from build123d import *

# Parameters (mm, degrees)
SKETCH_1_W      = 60
SKETCH_1_H      = 18
SKETCH_1_W_2    = 50
SKETCH_1_H_2    = 8
EXTRUDE_1_DEPTH = 50
SKETCH_2_W      = 50
SKETCH_2_H      = 8
EXTRUDE_2_DEPTH = 0.5


with BuildPart() as part:
    # 스케치1 → 보스-돌출1 (new body)
    with BuildSketch(Plane.XY):
        with Locations((25, 4)):
            Rectangle(SKETCH_1_W, SKETCH_1_H)
        with Locations((25, 4)):
            Rectangle(SKETCH_1_W_2, SKETCH_1_H_2, mode=Mode.SUBTRACT)
    extrude(amount=EXTRUDE_1_DEPTH)

    # 스케치2 → 보스-돌출2 (add, symmetric)
    with BuildSketch(Plane.XY.offset(25)):
        with Locations((25, 4)):
            Rectangle(SKETCH_2_W, SKETCH_2_H)
    extrude(amount=EXTRUDE_2_DEPTH, both=True)


solid = part.part
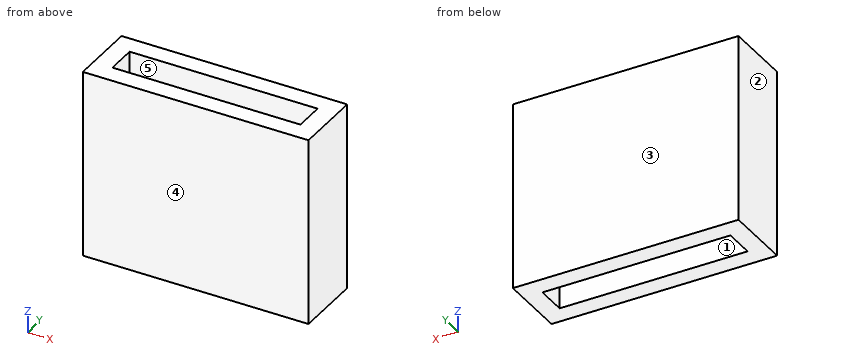
Geometry check sheet. Reference: the model listing, model coordinates, mm. Face numbers are marked on the shaded views. A direction names the side the tool comes from. Round coordinates to 2 decimals unless told otherwise and drop trailing zeros. Loops run counter-clockwise (first coordinate to the right, second up) from the corner with the lowest first, then second, coordinate; pieces in that order, holes last.
Item 1: Cross-section at B-B on y = 5.75. Record the boundary of the cut face in (x, z), then the cut area to 3 significant figures.
Item 2: Cross-section at A-A on z = 10. Record the boundary of the cut face in (x, y).
Item 3: Thickness scan on line 1 (Y direction, x = 45.5, z = 44.5); line 2 (X direction, y = 4, z = 32); line 3 (Z direction, x = 2.5, y = 1.25). Record the ranges inside material, lowest first.
Item 4: Mould release check, pull along Y, two halves, no side actions. Record for the marked faces 1, 2 and 3: pulls with the +Y half, pulls with the -Y half, needs draft (parallel to the pull), parting line crosses it, or undercut.
Item 5: Cross-section at C-C on x = 8. Record the boundary of the cut face in (y, z).
Item 6: Gauge pin test, flat end, axial feed: pin 1 (2.5 mm diameter, centred on x = 15, y = 3, fed in from -Z). Record the tip position at first contact, or that the pin passes through.
Item 7: Access from +Z, -Z, +X, -X, +Y, -Y to the whole of each face (thin tool, end or side, straight path). Record for the marked faces 4 and 5.
Answer sheet:
1. outline: (-5, 0) - (0, 0) - (0, 24.5) - (50, 24.5) - (50, 0) - (55, 0) - (55, 50) - (50, 50) - (50, 25.5) - (0, 25.5) - (0, 50) - (-5, 50) - close
1. area: 550 mm2
2. outline: (-5, -5) - (55, -5) - (55, 13) - (-5, 13) - close; hole (0, 0) - (50, 0) - (50, 8) - (0, 8) - close
3. line 1: y = -5 to 0, 8 to 13
3. line 2: x = -5 to 0, 50 to 55
3. line 3: z = 24.5 to 25.5
4. face 1: undercut
4. face 2: needs draft
4. face 3: pulls with the +Y half
5. outline: (-5, 0) - (0, 0) - (0, 24.5) - (8, 24.5) - (8, 0) - (13, 0) - (13, 50) - (8, 50) - (8, 25.5) - (0, 25.5) - (0, 50) - (-5, 50) - close
6. pin 1: stops at z = 24.5
7. face 4: +Z, -Z, +X, -X, -Y
7. face 5: +Z
